Autodesk Inventor part; units mm, degrees
ref_plane "Plano inicial" through (0, 0, -23.5401) normal (0, 0, 1) x (1, 0, 0)
ref_plane "Plano final" through (0, 0, 2213.5401) normal (0, 0, 1) x (1, 0, 0)
ref_plane "Plano de trabajo4" through (25.4, 0, -25.4) normal (-0.7071, 0, -0.7071) x (-0.7071, 0, 0.7071)
ref_plane "Plano inicial" through (0, 0, -23.5401) normal (0, 0, 1) x (1, 0, 0)
ref_plane "Plano final" through (0, 0, 2213.5401) normal (0, 0, 1) x (1, 0, 0)
sketch "Boceto" plane through (0, 0, 0) normal (0, 0, 1) x (1, 0, 0)
  line L0 (-25.4, -19.05) -> (-25.4, 19.05)
  line L1 (-19.05, 25.4) -> (19.05, 25.4)
  line L2 (25.4, 19.05) -> (25.4, -19.05)
  line L3 (19.05, -25.4) -> (-19.05, -25.4)
  arc A0 (-25.4, -19.05) -> (-19.05, -25.4) centre (-19.05, -19.05) ccw
  arc A1 (-19.05, 25.4) -> (-25.4, 19.05) centre (-19.05, 19.05) ccw
  arc A2 (25.4, 19.05) -> (19.05, 25.4) centre (19.05, 19.05) ccw
  arc A3 (19.05, -25.4) -> (25.4, -19.05) centre (19.05, -19.05) ccw
  arc A4 (-19.05, 22.225) -> (-22.225, 19.05) centre (-19.05, 19.05) ccw
  line L4 (-19.05, 22.225) -> (19.05, 22.225)
  arc A5 (22.225, 19.05) -> (19.05, 22.225) centre (19.05, 19.05) ccw
  line L5 (22.225, 19.05) -> (22.225, -19.05)
  arc A6 (19.05, -22.225) -> (22.225, -19.05) centre (19.05, -19.05) ccw
  line L6 (19.05, -22.225) -> (-19.05, -22.225)
  arc A7 (-22.225, -19.05) -> (-19.05, -22.225) centre (-19.05, -19.05) ccw
  line L7 (-22.225, -19.05) -> (-22.225, 19.05)
  line L8 (0, 37.4012) -> (0, -37.4012) construction
  line L9 (-37.4012, 0) -> (37.4012, 0) construction
  dimension "d10" = 50.8
  dimension "d11" = 50.8
  dimension "d12" = 3.175
  dimension "d15" = 25.4
  dimension "d16" = 25.4
  dimension "d17" = 6.35
extrude "Cuerpo" add sketch "Boceto" along normal up to surface (2237.0803 mm away) from surface at -23.5401
sketch "Sketch3" plane through (0, 0, 0) normal (0, 0, 1) x (1, 0, 0)
  line L0 (0, 0) -> (10, 0)
ref_plane "Work Plane3" through (0, 0, 0) normal (0, -1, 0) x (1, 0, 0)
ref_plane "Plano de trabajo4" through (25.4, 0, -25.4) normal (-0.7071, 0, -0.7071) x (-0.7071, 0, 0.7071)
split "Dividir1" plane through (25.4, 0, -25.4) removes the side toward (-0.7071, 0, -0.7071)
ref_plane "Plano de trabajo5" through (0, -25.4, -25.4) normal (0, 0.7071, -0.7071) x (1, 0, 0)
split "Dividir2" plane through (0, -25.4, -25.4) removes the side toward (0, 0.7071, -0.7071)
ref_plane "Plano de trabajo6" through (25.4, 0, 2215.4) normal (-0.7071, 0, 0.7071) x (0.7071, 0, 0.7071)
split "Dividir3" plane through (25.4, 0, 2215.4) removes the side toward (-0.7071, 0, 0.7071)
ref_plane "Plano de trabajo7" through (0, -25.4, 2215.4) normal (0, 0.7071, 0.7071) x (1, 0, 0)
split "Dividir4" plane through (0, -25.4, 2215.4) removes the side toward (0, 0.7071, 0.7071)
sketch "Sketch4" plane through (0, 0, 0) normal (0, -1, 0) x (1, 0, 0)
  line L0 (-2, -23.5401) -> (12, -23.5401)
  line L1 (-2, 2213.5401) -> (12, 2213.5401)
  dimension "d19" = 2237.0803
equation "\"d10\" = G_H"
equation "\"d11\" = G_W"
equation "\"d12\" = G_T"
equation "\"d15\" = 0.5 * d10"
equation "\"d16\" = 0.5 * d11"
equation "\"d17\" = G_IR"
equation "\"d3\" = G_L"
equation "\"G_W\" = 50.8"
equation "\"G_H\" = 50.8"
equation "\"G_T\" = 3.175"
equation "\"G_IR\" = 6.35"
equation "\"G_L\" = d19"
equation "\"G_OFFSET_START\" = 23.54013"
equation "\"G_OFFSET_END\" = 23.54013"
equation "\"d13\" = -G_OFFSET_START"
equation "\"d14\" = G_OFFSET_END + B_L"
equation "\"B_L\" = 2190"
properties part number "AISC - 2 x 2 x 1/8 - 88,074" material "Acero, suave"
Here's how the part is built. I have some questions about the finished solid (model axes, mm). A direction names the side the tool comes from. Coordinates: 2 decimals unless noted, no trailing zeros. Write each loop counter-clockwise with the first axis right and the second up, starting at its lowest first coordinate (ties: lowest second). Pieces come first, ordered by that corner, then holes. Notation, with made-up numbers: (52, 23) - (106, 23) arc R11 ccw to (106, 43) - close; hole circle Ø3 at (2.25, 71.5). An arc over 180 degrees is marked (long way). Use one line per item in the form item = value.
1) I need wall thicknesses on line 1 (X direction, y = -15, z = 120.5) (3 decimals); line 2 (X direction, y = 20, z = 428). Which ranges of each line are inside material? Lowest first, please.
Solved:
line_1 = -25.4 to -22.225, 22.225 to 25.4
line_2 = -25.33 to -22.08, 22.08 to 25.33
2) Suppose I cut it at C-C, the plane z = 1909. Write out the boundary of the cut face in (x, y) (3 decimals).
Solved:
outline = (-25.4, -19.05) arc R6.35 ccw to (-19.05, -25.4) - (19.05, -25.4) arc R6.35 ccw to (25.4, -19.05) - (25.4, 19.05) arc R6.35 ccw to (19.05, 25.4) - (-19.05, 25.4) arc R6.35 ccw to (-25.4, 19.05) - close; hole (-22.225, -19.05) arc R3.175 ccw to (-19.05, -22.225) - (19.05, -22.225) arc R3.175 ccw to (22.225, -19.05) - (22.225, 19.05) arc R3.175 ccw to (19.05, 22.225) - (-19.05, 22.225) arc R3.175 ccw to (-22.225, 19.05) - close
3) Suppose I cut it at B-B, the plane x = -6.5. Write out the boundary of the cut face in (y, z) (3 decimals), plus the area to 3 significant figures.
Solved:
outline = (-25.4, 6.5) - (-22.225, 6.5) - (-22.225, 2183.5) - (-25.4, 2183.5) - close; (22.225, 22.225) - (25.4, 25.4) - (25.4, 2164.6) - (22.225, 2167.775) - close
area = 13,700 mm2
4) Suppose I cut it at A-A, the plane y = -10. Write out the boundary of the cut face in (x, z) (3 decimals).
Solved:
outline = (-25.4, 25.4) - (-22.225, 22.225) - (-22.225, 2167.775) - (-25.4, 2164.6) - close; (22.225, -10) - (25.4, -10) - (25.4, 2200) - (22.225, 2200) - close
5) Thinking about a two-plate mould opening in Y: for faces 3 (the flat face through (25.4, 0, 1079)), 4 (the flat face through (23, 12, 2178)), 5 (the flat face through (0, -25.4, 1079)), 6 (the flat face through (-22.225, 0, 1080)), which applies, released by +Y, released by -Y, zero draft, split by the parting line, or undercut?
Solved:
face_3 = zero draft
face_4 = released by +Y
face_5 = released by -Y
face_6 = undercut
6) On a 3-axis mill with a long thin cutter (end or side, diameter ignored), from which of +Z, -Z, +X, -X, +Y, -Y can I reach the whole of each face in a straight line? I mean faces 1 (the flat face through (-25.4, 0, 1080)), 2 (the flat face through (0, -22.225, 1079)). Say none if no direction works.
Solved:
face_1 = +Z, -Z, -X, +Y, -Y
face_2 = +Z, -Z
